Part model, mm, in its own coordinate system. Face numbers are marked on the shaded views. A direction names the side the tool comes from. Give positions to 0.01 mm unless a question says otherwise; leave off trailing zeros. Write each loop counter-clockwise with the first axis right and the second up, starting at its lowest first coordinate (ties: lowest second). Pieces come first, ordered by that corner, then holes. Notation, with made-up numbers: (78, 55) - (132, 55) arc R38 ccw to (132, 94) - close; hole circle Ø2 at (41, 0). An arc over 180 degrees is marked (long way). Answer in a Markdown table with one row per item. Add a question column.
1. Band-saw the part on A-A on y = -1.55. Write the cut outline in (x, z), plus the area to 3 significant figures.
2. Pull direction Y, two halves, no side cores. Call the marked faces 4, 5 and 6: released by +Y, released by -Y, zero draft, split by the parting line, or undercut.
3. Band-saw the part on B-B on z = 4. Write the cut outline in (x, y), plus the area to 3 significant figures.
4. Band-saw the part on C-C on z = -7.75. Write the cut outline in (x, y), plus the area to 3 significant figures.
5. Which spindle directions (+Z, -Z, +X, -X, +Y, -Y) get a long thin tool onto all of the face, cutting with end or side? Do the marked faces 1, 2 and 3. Say none if no direction does.
6. Drop flat-ended pins along their axis: pin 1 Ø1.2 at (x, y) = (0, 0) entering from -Z; pin 2 Ø0.6 at (x, y) = (0, 0) entering from +Z. Give the stop position or say it passes through.
7. Probe line 1 along Z through (x, y) = (-0.5, -1.4); line 2 along X through (y, z) = (-0.95, -6.5); line 3 along Y through (x, z) = (0, -5.45). List the from-to ranges inside material, lowest first.
Autodesk Fusion 360 part; units mm, degrees
sketch "Sketch1" plane through (0, 0, 0) normal (0, 0, 1) x (1, 0, 0)
  line L0 (3, -2.5) -> (-3, -2.5)
  line L1 (-3, -2.5) -> (-3, 2.5)
  line L2 (-3, 2.5) -> (3, 2.5)
  line L3 (3, 2.5) -> (3, -2.5)
  line L4 (3, -2.5) -> (-3, 2.5) construction
  line L5 (-3, -2.5) -> (3, 2.5) construction
  dimension "dWidth" = 6
  dimension "d2" = 5
extrude "Extrude1" add sketch "Sketch1" along normal blind 10.5
sketch "Sketch2" plane through (0, 0, 10.5) normal (0, 0, 1) x (1, 0, 0)
  line L0 (3, 2.5) -> (-3, 2.5)
  line L1 (-3, 2.5) -> (-3, -2.5)
  line L2 (-3, -2.5) -> (3, -2.5)
  line L3 (3, -2.5) -> (3, 2.5)
  circle A0 centre (0, 0) radius 1
  dimension "d5" = 2
extrude "Extrude2" cut sketch "Sketch2" against normal blind 7 contours A0
ref_plane "WorkPlane1" through (0, 0, 8) normal (0, 0, 1) x (1, 0, 0)
sketch "Sketch3" plane through (0, 0, 8) normal (0, 0, 1) x (1, 0, 0)
  line L0 (2, -2.16) -> (-2, -2.16) construction
  line L1 (-2, -2.16) -> (-2, 2.16) construction
  line L2 (-2, 2.16) -> (2, 2.16) construction
  line L3 (2, 2.16) -> (2, -2.16) construction
  line L4 (2, -2.16) -> (-2, 2.16) construction
  line L5 (-2, -2.16) -> (2, 2.16) construction
  line L6 (-2, 0) -> (2, 0) construction
  line L7 (2, 1.1258) -> (2, -1.1258)
  line L8 (-2, 1.1258) -> (-2, -1.1258)
  line L9 (0, 2.16) -> (0, -2.16) construction
  line L10 (-2, 1.1258) -> (0, 2.16)
  line L11 (2, 1.1258) -> (0, 2.16)
  line L12 (-2, -1.1258) -> (0, -2.16) construction
  line L13 (0, -2.16) -> (2, -1.1258) construction
  line L14 (-2, -1.1258) -> (-2, -2.5)
  line L15 (-2, -2.5) -> (2, -2.5)
  line L16 (2, -2.5) -> (2, -1.1258)
  line L17 (3, -2.5) -> (-3, -2.5)
  dimension "d9" = 4
  dimension "d10" = 4.32
extrude "Extrude3" cut sketch "Sketch3" against normal blind 1.6
fillet "Fillet1" radius 0.75 2 edges at (-3, 2.5, 5.25) (3, 2.5, 5.25)
chamfer "Chamfer2" distance 0.5 angle 75 2 edges at (3, -0.375, 10.5) (-3, -0.375, 10.5) measured on face at (-2.3296, -0.2997, 10.5) measured on face at (-2.3296, -0.2997, 10.5)
mirror "Mirror2" about plane through (0, 0, 0) normal (0, 0, 1) of bodies 1 merged
properties part number "Configuration 2"
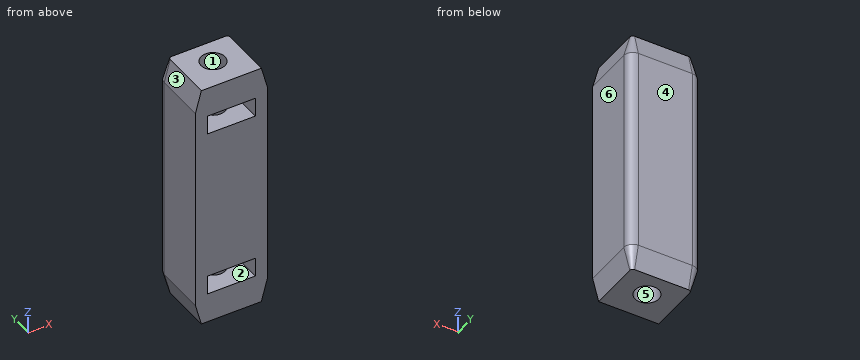
Values:
| question | item | result |
|---|---|---|
| 1 | outline | (-3, -8.63) - (-2.5, -10.5) - (2.5, -10.5) - (3, -8.63) - (3, 8.63) - (2.5, 10.5) - (-2.5, 10.5) - (-3, 8.63) - close; hole (-2, -8) - (2, -8) - (2, -6.4) - (-2, -6.4) - close; hole (-2, 6.4) - (2, 6.4) - (2, 8) - (-2, 8) - close |
| 1 | area | 111 mm² |
| 2 | face 4 | released by +Y |
| 2 | face 5 | undercut |
| 2 | face 6 | zero draft |
| 3 | outline | (-3, -2.5) - (3, -2.5) - (3, 1.75) arc R0.75 ccw to (2.25, 2.5) - (-2.25, 2.5) arc R0.75 ccw to (-3, 1.75) - close; hole circle Ø2 at (0, 0) |
| 3 | area | 26.6 mm² |
| 4 | outline | (-3, -2.5) - (-2, -2.5) - (-2, 1.13) - (0, 2.16) - (2, 1.13) - (2, -2.5) - (3, -2.5) - (3, 1.75) arc R0.75 ccw to (2.25, 2.5) - (-2.25, 2.5) arc R0.75 ccw to (-3, 1.75) - close |
| 4 | area | 13.2 mm² |
| 5 | face 1 | +Z |
| 5 | face 2 | -Y |
| 5 | face 3 | +Z, -X, +Y, -Y |
| 6 | pin 1 | stops at z = -3.5 |
| 6 | pin 2 | stops at z = 3.5 |
| 7 | line 1 | z = -10.5 to -8, -6.4 to 6.4, 8 to 10.5 |
| 7 | line 2 | x = -3 to -2, 2 to 3 |
| 7 | line 3 | y = -2.5 to -1, 1 to 2.5 |
